```python
from build123d import *

# Parameters (mm, degrees)
SALIENTE_EXTRUIR1_DEPTH = 50
CROQUIS2_R              = 5
CORTAR_EXTRUIR1_DEPTH   = 10


with BuildPart() as part:
    # Croquis1 → Saliente-Extruir1 (new body)
    with BuildSketch(Plane.XY):
        Polygon((0, 24.535031847), (14.422205102, 0.535031847), (0, -23.464968153), (-14.422205102, 0.535031847), align=None)
    extrude(amount=SALIENTE_EXTRUIR1_DEPTH)

    # Croquis2 → Cortar-Extruir1 (cut)
    with BuildSketch(Plane(origin=(0, 0, 0), x_dir=(-1, 0, 0), z_dir=(0, 0, -1))):
        Circle(CROQUIS2_R)
    extrude(amount=-CORTAR_EXTRUIR1_DEPTH, mode=Mode.SUBTRACT)


solid = part.part
```
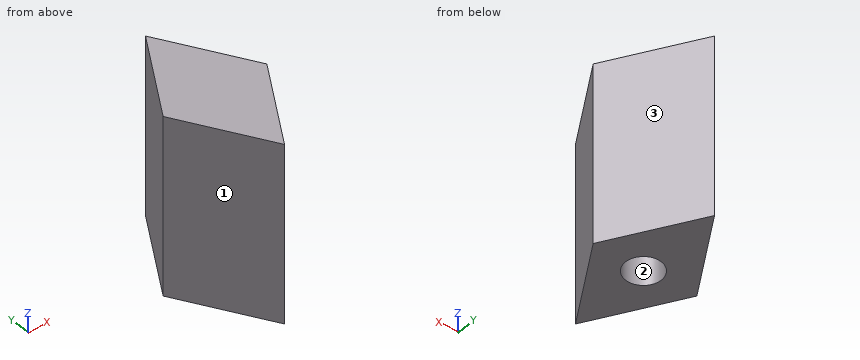
CAD build for the part. Positions are in the model's coordinates, mm. Face numbers are marked on the shaded views. Round coordinates to 2 decimals unless told otherwise and drop trailing zeros. Order: outer loops, then holes, each group sorted by start corner. A loop starts at its lowest first (then second) coordinate and runs counter-clockwise, first axis right, second up. Notation, with made-up numbers: (11.25, 15.5) -> (27.25, 15.5) arc R21 ccw to (27.25, 54.5) -> close; hole circle Ø5 at (-30.75, -33). An arc over 180 degrees is marked (long way). Write item = value, one per line.
(1) Drill centre lines: L1, parallel to X at y = 15.5, z = 13.5; L2, parallel to Y at x = -3.5, z = 43.5; L3, parallel to X at y = 13, z = 40.5. Where is each one in solid material? Low to high.
Answers follow:
L1 = -5.43 to 5.43
L2 = -17.64 to 18.71
L3 = -6.93 to 6.93
(2) Pull direction Y, two halves, no side cores. Call the marked faces 1, 2 and 3: +Y half, -Y half, draft (parallel to the pull), parting line (faces both ways), or undercut.
Answers follow:
face_1 = -Y half
face_2 = undercut
face_3 = +Y half
(3) Cut at D-D (y = -3). Write the cut outline in (x, z), plus the area to 3 significant figures.
Answers follow:
outline = (-12.3, 0) -> (-4, 0) -> (-4, 10) -> (4, 10) -> (4, 0) -> (12.3, 0) -> (12.3, 50) -> (-12.3, 50) -> close
area = 1,150 mm²
(4) Cut at A-A (z = 7). Write the cut outline in (x, y).
Answers follow:
outline = (-14.42, 0.54) -> (0, -23.46) -> (14.42, 0.54) -> (0, 24.54) -> close; hole circle Ø10 at (0, 0)
(5) Cut at B-B (x = 3.5). Write the cut outline in (y, z), plus the area to 3 significant figures.
Answers follow:
outline = (-17.64, 0) -> (-3.57, 0) -> (-3.57, 10) -> (3.57, 10) -> (3.57, 0) -> (18.71, 0) -> (18.71, 50) -> (-17.64, 50) -> close
area = 1,750 mm²
(6) Cut at C-C (z = 16). Write the cut outline in (x, y), plus the area to 3 significant figures.
Answers follow:
outline = (-14.42, 0.54) -> (0, -23.46) -> (14.42, 0.54) -> (0, 24.54) -> close
area = 692 mm²
(7) Flat gauge pins, fed straight in: P1, Ø12, axis at x = -0.5, z = 23.5, coming from the -Y side; P2, Ø1, axis at y = 12.5, z = 32, coming from the -X side; P3, Ø10, axis at x = -10, z = 13, coming from the +Y side. Where does each tip first touch, or does it go through?
Answers follow:
P1 = -23.46
P2 = -7.53
P3 = 16.21
